from build123d import *

# Parameters (mm, degrees)
F1_DEPTH = 9
F3_R     = 3
F4_DEPTH = 16
F2_R     = 3
F5_DEPTH = 15.325


with BuildPart() as f1:
    # F0 (on Top) → F1 (new body)
    with BuildSketch(Plane.XY):
        Polygon((8, 13.089484), (0, 13.089484), (-8, 13.089484), (-8, 4.089484), (-4.5, 4.041417), (-4.5, -3.731445), (0, -3.731445), (4.5, -3.731445), (4.5, 4.089484), (8, 4.089484), align=None)
    extrude(amount=F1_DEPTH)

    # F3 (on face) → F4 (cut)
    with BuildSketch(Plane.YZ.offset(8)):
        with Locations((8.589484, 4.5)):
            Circle(F3_R)
    extrude(amount=-F4_DEPTH, mode=Mode.SUBTRACT)

    # F2 (on face) → F5 (cut)
    with BuildSketch(Plane.XZ.offset(3.731445)):
        with Locations((0, 4.5)):
            Circle(F2_R)
    extrude(amount=-F5_DEPTH, mode=Mode.SUBTRACT)


solid = f1.part
Build history of the part. All positions in model axes, mm. A direction names the side the tool comes from. Give positions to 0.01 mm unless a question says otherwise; leave off trailing zeros. Write each loop counter-clockwise with the first axis right and the second up, starting at its lowest first coordinate (ties: lowest second). Pieces come first, ordered by that corner, then holes. Notation, with made-up numbers: (80, 61) - (109, 61) arc R12 cw to (109, 80) - close; hole circle Ø6 at (0.25, -5.5). An arc over 180 degrees is marked (long way). Use one line per item in the form item = value. Start each with the question number.
1. Band-saw the part on D-D on z = 1.25. Write the cut outline in (x, y), plus the area to 3 significant figures.
2. Probe line 1 (Y direction, x = -3.75, z = 4.5); line 2 (Z direction, x = 0, y = 9.3); line 3 (X direction, y = 1.75, z = 4.5). List the from-to ranges inside material, lowest first. Write a range as [from, to].
3. Band-saw the part on A-A on z = 4.5. Count the separate pieces of the cut face and the enclosed holes in it, plus the area to 3 significant figures.
4. Band-saw the part on B-B on x = 5. Write the cut outline in (y, z).
5. Two-plate mould, pull along X, no slides. Class faces 4 (the face through (0, 11.594, 5)), 5 (the face through (0, -3.731, 1)), 6 (the face through (4.5, 0, 4)): released by +X, released by -X, zero draft, split by the parting line, or undercut.
6. 3-axis set-ups, long thin cutter, end or side, ignore diameter. For faces 1 (the face through (-4.5, 0, 4)), 2 (the face through (1.5, 10.6, 1.9)), 3 (the face through (6, 4.089, 4)): which of +Z, -Z, +X, -X, +Y, -Y reach the whole face in a straight line?
7. Drop flat-ended pins along their axis: pin 1 Ø3 at (x, z) = (0, 7) entering from -Y; pin 2 Ø2 at (y, z) = (-1.5, 3) entering from -X; pin 3 Ø4 at (x, z) = (7, 6.5) entering from -Y. Give the stop position or say it passes through.
8. Band-saw the part on C-C on y = 0.75. Write the cut outline in (x, z), plus the area to 3 significant figures.
Conclusion:
q1.outline = (-8, 4.09) - (-4.5, 4.04) - (-4.5, -3.73) - (4.5, -3.73) - (4.5, 4.09) - (8, 4.09) - (8, 13.09) - (-8, 13.09) - close
q1.area = 214 mm²
q2.line_1 = [-3.73, 5.59], [11.59, 13.09]
q2.line_2 = [0, 1.5], [7.5, 9]
q2.line_3 = [-4.5, -3], [3, 4.5]
q3.separate_pieces = 3
q3.enclosed_holes = 0
q3.area = 62.5 mm²
q4.outline = (4.09, 0) - (13.09, 0) - (13.09, 9) - (4.09, 9) - close; hole circle Ø6 at (8.59, 4.5)
q5.face_4 = undercut
q5.face_5 = zero draft
q5.face_6 = released by +X
q6.face_1 = +Z, -Z, -X, -Y
q6.face_2 = -Y
q6.face_3 = +Z, -Z, +X, -Y
q7.pin_1 = -3.73
q7.pin_2 = -4.5
q7.pin_3 = 4.09
q8.outline = (-4.5, 0) - (4.5, 0) - (4.5, 9) - (-4.5, 9) - close; hole circle Ø6 at (0, 4.5)
q8.area = 52.7 mm²
